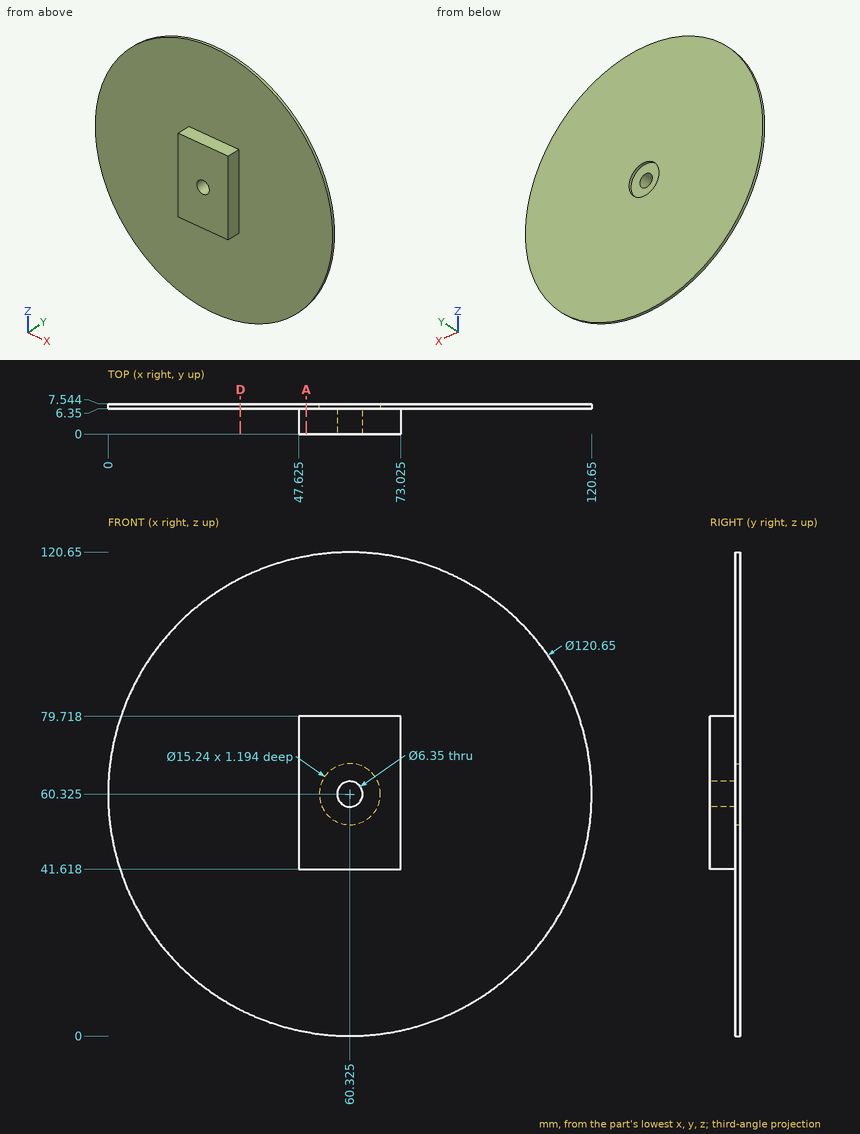
For this review, use the dimensioned drawing (mm, ordinates from the lowest corner) and the shaded views. Round coordinates to 2 decimals unless told otherwise and drop trailing zeros. Write each loop counter-clockwise with the first axis right and the second up, starting at its lowest first coordinate (ties: lowest second). Pieces come first, ordered by that corner, then holes. Notation, with made-up numbers: (-5.75, 61.25) - (17.25, 61.25) arc R23 ccw to (17.25, 70.25) - close; hole circle Ø10 at (69.25, 25.5). An arc over 180 degrees is marked (long way). Answer as a JSON object with one key per item and string values.
1. For pin 1 Ø3 at (y, z) = (4.5, 68.5) entering from +X (3 decimals); pin 2 Ø3 at (x, y) = (62.5, 4) entering from -Z; pin 3 Ø7.5 at (x, z) = (63, 61) entering from +Y, all flat-tipped, find the tip position at first contact; note any pin that passes through.
Response values:
{"pin 1": "stops at x = 73.025", "pin 2": "stops at z = 41.62", "pin 3": "stops at y = 6.35"}
2. We need section D-D on x = 33. Give the boundary of the cut face in (y, z).
Response values:
{"outline": "(6.35, 6.54) - (7.54, 6.54) - (7.54, 114.11) - (6.35, 114.11) - close"}
3. We need section A-A on x = 49.5. Give the boundary of the cut face in (y, z).
Response values:
{"outline": "(0, 41.62) - (6.35, 41.62) - (6.35, 0.98) - (7.54, 0.98) - (7.54, 119.67) - (6.35, 119.67) - (6.35, 79.72) - (0, 79.72) - close"}
4. To check wall thickness, follow line 1 along Z through (x, y) = (54, 3.75); line 2 along X through (y, z) = (1.25, 60.5) (1 decimal); line 3 along Y through (x, z) = (21, 52). State the ranges of each line that lie inside material, in increasing order.
Response values:
{"line 1": "z = 41.62 to 79.72", "line 2": "x = 47.6 to 57.2, 63.5 to 73", "line 3": "y = 6.35 to 7.54"}
